```python
from build123d import *

# Parameters (mm, degrees)
PAD_DEPTH       = 42.5
PAD001_DEPTH    = 26
PAD002_DEPTH    = 73
PAD003_DEPTH    = 8.5
SKETCH004_R     = 1.75
POCKET_DEPTH    = 5
SKETCH005_R     = 1.75
POCKET001_DEPTH = 5


with BuildPart() as part:
    # Sketch → Pad (new body, symmetric)
    with BuildSketch(Plane.XZ):
        with BuildLine():
            Line((-35.75, -35), (-37.75, -35))
            ThreePointArc((-38.25, -34.5), (-38.103553, -34.853553), (-37.75, -35))
            Line((-38.25, -34.5), (-38.25, -0.5))
            ThreePointArc((-37.75, 0), (-38.103553, -0.146447), (-38.25, -0.5))
            Line((-37.75, 0), (37.75, 0))
            ThreePointArc((38.25, -0.5), (38.103553, -0.146447), (37.75, 0))
            Line((38.25, -0.5), (38.25, -6.5))
            Line((38.25, -6.5), (38.05, -6.5))
            Line((38.05, -6.5), (38.05, -0.5))
            ThreePointArc((38.05, -0.5), (37.962132, -0.287868), (37.75, -0.2))
            Line((37.75, -0.2), (-37.75, -0.2))
            ThreePointArc((-37.75, -0.2), (-37.962132, -0.287868), (-38.05, -0.5))
            Line((-38.05, -0.5), (-38.05, -34.5))
            ThreePointArc((-38.05, -34.5), (-37.962132, -34.712132), (-37.75, -34.8))
            Line((-37.75, -34.8), (-35.75, -34.8))
            Line((-35.75, -34.8), (-35.75, -35))
        make_face()
    extrude(amount=PAD_DEPTH, both=True)

    # Sketch001 (on Face15 of Pad) → Pad001 (join)
    with BuildSketch(Plane(origin=(0, 0, -1), x_dir=(-1, 0, 0), z_dir=(0, 0, 1))):
        with BuildLine():
            ThreePointArc((38.25, 42.5), (38.103553, 42.853553), (37.75, 43))
            Line((37.75, 43), (28.75, 43))
            Line((28.75, 43), (28.75, 42.8))
            Line((28.75, 42.8), (37.75, 42.8))
            ThreePointArc((38.05, 42.5), (37.962132, 42.712132), (37.75, 42.8))
            Line((38.05, 42.5), (38.25, 42.5))
        make_face()
        with BuildLine():
            ThreePointArc((37.75, -43), (38.103553, -42.853553), (38.25, -42.5))
            Line((38.05, -42.5), (38.25, -42.5))
            ThreePointArc((37.75, -42.8), (37.962132, -42.712132), (38.05, -42.5))
            Line((37.75, -42.8), (28.75, -42.8))
            Line((28.75, -42.8), (28.75, -43))
            Line((28.75, -43), (37.75, -43))
        make_face()
    extrude(amount=-PAD001_DEPTH)

    # Sketch002 (on Face9 of Pad001) → Pad002 (join)
    with BuildSketch(Plane(origin=(-37.25, 0, 0), x_dir=(0, 0, -1), z_dir=(-1, 0, 0))):
        with BuildLine():
            ThreePointArc((0.5, 43.2), (0.146447, 43.053553), (0, 42.7))
            Line((0, 42.7), (0, 42.5))
            Line((0, 42.5), (0.2, 42.5))
            Line((0.2, 42.5), (0.2, 42.7))
            ThreePointArc((0.5, 43), (0.287868, 42.912132), (0.2, 42.7))
            Line((0.5, 43), (10.5, 43))
            Line((10.5, 43), (10.5, 43.2))
            Line((10.5, 43.2), (0.5, 43.2))
        make_face()
        with BuildLine():
            ThreePointArc((0, -42.7), (0.146447, -43.053553), (0.5, -43.2))
            Line((4.5, -43.2), (0.5, -43.2))
            Line((4.5, -43), (4.5, -43.2))
            Line((0.5, -43), (4.5, -43))
            ThreePointArc((0.2, -42.7), (0.287868, -42.912132), (0.5, -43))
            Line((0.2, -42.5), (0.2, -42.7))
            Line((0, -42.5), (0.2, -42.5))
            Line((0, -42.7), (0, -42.5))
        make_face()
    extrude(amount=-PAD002_DEPTH)

    # Sketch003 (on Face38 of Pad002) → Pad003 (join)
    with BuildSketch(Plane(origin=(-28.75, 0, 0), x_dir=(0, 0, 1), z_dir=(1, 0, 0))):
        with BuildLine():
            ThreePointArc((-28.3, 44.3), (-27.919239, 43.380761), (-27, 43))
            Line((-27, 43), (-27, 42.8))
            ThreePointArc((-28.5, 44.3), (-28.06066, 43.23934), (-27, 42.8))
            Line((-28.5, 61.3), (-28.5, 44.3))
            Line((-28.3, 61.3), (-28.5, 61.3))
            Line((-28.3, 44.3), (-28.3, 61.3))
        make_face()
    extrude(amount=-PAD003_DEPTH)

    # Sketch004 (on Face36 of Pad003) → Pocket (cut)
    with BuildSketch(Plane(origin=(0, 43, 0), x_dir=(1, 0, 0), z_dir=(0, 1, 0))):
        with Locations((-32.75, 15)):
            Circle(SKETCH004_R)
    extrude(amount=-POCKET_DEPTH, mode=Mode.SUBTRACT)

    # Sketch005 (on Face59 of Pocket) → Pocket001 (cut)
    with BuildSketch(Plane(origin=(0, 0, -28.3), x_dir=(-1, 0, 0), z_dir=(0, 0, 1))):
        with Locations((33.25, 56.8)):
            Circle(SKETCH005_R)
    extrude(amount=-POCKET001_DEPTH, mode=Mode.SUBTRACT)


solid = part.part
```
Work out the finished part from the listing and answer in its coordinate system (mm). A direction names the side the tool comes from. Give positions to 0.01 mm unless a question says otherwise; leave off trailing zeros. Order: outer loops, then holes, each group sorted by start corner. A loop starts at its lowest first (then second) coordinate and runs counter-clockwise, first axis right, second up.
1. Section C-C, the plane y = -56.8 is taken. Determine the outline of the cut face in (x, z).
Result sheet:
outline: (-37.25, -28.5) - (-35, -28.5) - (-35, -28.3) - (-37.25, -28.3) - close; (-31.5, -28.5) - (-28.75, -28.5) - (-28.75, -28.3) - (-31.5, -28.3) - close
2. Section A-A, the plane x = 24.5 is taken. Determine the outline of the cut face in (y, z).
Result sheet:
outline: (-43.2, -10.5) - (-43, -10.5) - (-43, -0.5) arc R0.3 cw to (-42.7, -0.2) - (42.7, -0.2) arc R0.3 cw to (43, -0.5) - (43, -4.5) - (43.2, -4.5) - (43.2, -0.5) arc R0.5 ccw to (42.7, 0) - (-42.7, 0) arc R0.5 ccw to (-43.2, -0.5) - close
3. Section D-D, the plane x = -33.25 is taken. Give the number of separate pieces and of enclosed holes in the cut face, and give its area (3 significant figures).
Result sheet:
separate pieces: 3
enclosed holes: 0
area: 33.0 mm2
4. Each of these flat-tipped pins is pushed along its axis until it touches: P1, Ø4.5, axis at x = -32.75, z = -15, coming from the +Y side; P2, Ø4, axis at y = -46.5, z = -13, coming from the -X side; P3, Ø1, axis at x = -37, y = 13.5, coming from the +Z side; P4, Ø0.8, axis at y = 43, z = -3, coming from the +X side. Where does it stop, or does it pass through?
Result sheet:
P1: stops at y = 43
P2: passes through
P3: stops at z = 0
P4: stops at x = 35.75
5. For faces 4 (the flat face through (-33, -53, -28.3)), 5 (the flat face through (-1, -1, 0)), 6 (the flat face through (38.05, -1, -4)), 7 (the flat face through (-33, -42.8, -14)), 8 (the flat face through (-38.25, -1, -18)), determine the directions among +Z, -Z, +X, -X, +Y, -Y from which every point of the face is accessible in a straight line to the end or side of a thin tool.
Result sheet:
face 4: +Z, +X, -X, -Y
face 5: +Z, +X, -X, +Y, -Y
face 6: -Z, +Y, -Y
face 7: -Z, +X
face 8: +Z, -Z, -X, +Y, -Y
6. Section B-B, the plane z = -3 is taken. Determine the outline of the cut face in (x, y).
Result sheet:
outline: (-38.25, -42.5) arc R0.5 ccw to (-37.75, -43) - (-37.25, -43) - (-37.25, -43.2) - (35.75, -43.2) - (35.75, -43) - (-28.75, -43) - (-28.75, -42.8) - (-37.75, -42.8) arc R0.3 cw to (-38.05, -42.5) - (-38.05, 42.5) arc R0.3 cw to (-37.75, 42.8) - (-28.75, 42.8) - (-28.75, 43) - (35.75, 43) - (35.75, 43.2) - (-37.25, 43.2) - (-37.25, 43) - (-37.75, 43) arc R0.5 ccw to (-38.25, 42.5) - close; (38.05, -42.5) - (38.25, -42.5) - (38.25, 42.5) - (38.05, 42.5) - close
7. Straight lines are drawn through the part: L1, parallel to X at y = 42.9, z = -15; L2, parallel to X at y = -56.8, z = -28.4; L3, parallel to X at y = 7, z = -10.5. For each, find the intervals that lie inside material, in ascending order.
Result sheet:
L1: x = -38.05 to -34.5, -31 to -28.75
L2: x = -37.25 to -35, -31.5 to -28.75
L3: x = -38.25 to -38.05
8. The mould has two halves that part along Y. Classify faces 1 (the flat face through (-38.05, -1, -17)), 2 (the flat face through (-1, -43.2, -6)), 3 (the flat face through (38.25, -1, -3)): released by +Y, released by -Y, zero draft, split by the parting line, or undercut.
Result sheet:
face 1: undercut
face 2: released by -Y
face 3: zero draft
